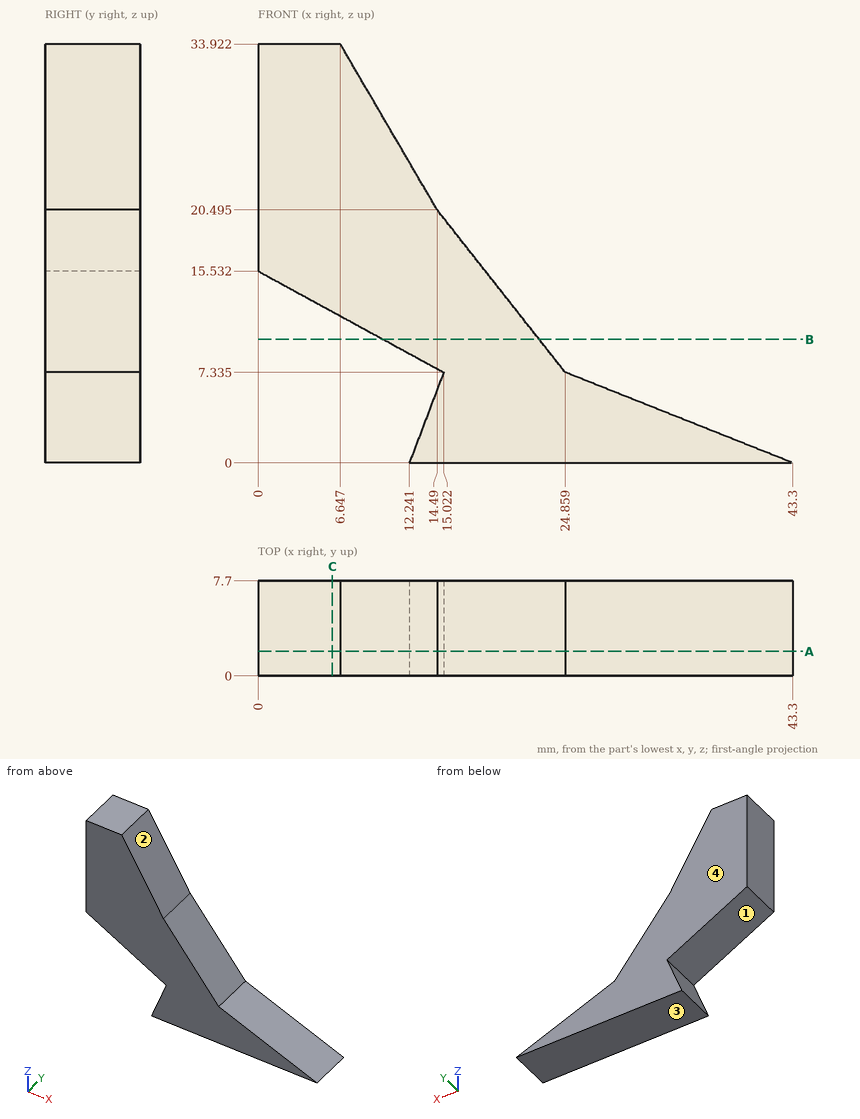
Could you check a few things on this drawing? It's one solid part, dimensions in mm from its lowest x, y, z. Round coordinates to 2 decimals unless told otherwise and drop trailing zeros. Loops run counter-clockwise (first coordinate to the right, second up) from the corner with the lowest first, then second, coordinate; pieces in that order, holes last. Notation, with made-up numbers: M 35.5,21.25 L 58.5,21.25 A12 ccw 58.5,33.25 Z; hole C -18,-23.75 d3. An arc over 180 degrees is marked long. Write item = value, one per line. Start each with the question number.
(1) Suppose I cut it at C-C on x = 6. Write out the boundary of the cut face in (y, z), plus the area to 3 significant figures.
(2) If we mould it in two halves opening along Z, with no side actions, what happens to the marked faces 1, 2, 3 and 4? For each: released by +Z, released by -Z, zero draft, split by the parting line, or undercut.
(3) Suppose I cut it at B-B on z = 10. Write out the boundary of the cut face in (x, y).
(4) Suppose I cut it at A-A on y = 2. Write out the boundary of the cut face in (x, z) (1 decimal), plus the area to 3 significant figures.
(5) I need wall thicknesses on line 1 along X through (y, z) = (1.25, 11) (1 decimal); line 2 along X through (y, z) = (7, 20); line 3 along Z through (x, y) = (35.5, 5.75). Which ranges of each line are inside material? Lowest first, please.
Answer block:
q1.outline = M 0,12.26 L 7.7,12.26 L 7.7,33.92 L 0,33.92 Z
q1.area = 167 mm²
q2.face_1 = undercut
q2.face_2 = released by +Z
q2.face_3 = released by -Z
q2.face_4 = zero draft
q3.outline = M 10.14,0 L 22.76,0 L 22.76,7.7 L 10.14,7.7 Z
q4.outline = M 0,15.5 L 15,7.3 L 12.2,0 L 43.3,0 L 24.9,7.3 L 14.5,20.5 L 6.6,33.9 L 0,33.9 Z
q4.area = 489 mm²
q5.line_1 = 8.3 to 22
q5.line_2 = 0 to 14.88
q5.line_3 = 0 to 3.1
